```python
from build123d import *

# Parameters (mm, degrees)
SKETCH1_W                        = 12.7
SKETCH1_H                        = 12.7
BOSS_EXTRUDE1_DEPTH              = 72
F_10_24_TAPPED_HOLE1_D           = 3.7973
F_10_24_TAPPED_HOLE2_D           = 3.7973
M6X1_0_TAPPED_HOLE2_D            = 5
M6X1_0_TAPPED_HOLE2_DEPTH        = 20.32
M6X1_0_TAPPED_HOLE2_CSINK_D      = 6.05
M6X1_0_TAPPED_HOLE2_CSINK_ANGLE  = 90
M6X1_0_TAPPED_HOLE2_TIP          = 1.502151548
F_10_24_TAPPED_HOLE3_D           = 3.7973
F_10_24_TAPPED_HOLE3_DEPTH       = 20.574
F_10_24_TAPPED_HOLE3_CSINK_D     = 5.0673
F_10_24_TAPPED_HOLE3_CSINK_ANGLE = 90
F_10_24_TAPPED_HOLE3_TIP         = 1.140824014
LPATTERN1_COUNT                  = 2
LPATTERN1_PITCH                  = 24
LPATTERN2_COUNT                  = 2
LPATTERN2_PITCH                  = 24


with BuildPart() as part:
    # Sketch1 → Boss-Extrude1 (new body)
    with BuildSketch(Plane(origin=(0, 0, 0), x_dir=(0, 0, -1), z_dir=(1, 0, 0))):
        Rectangle(SKETCH1_W, SKETCH1_H)
    extrude(amount=BOSS_EXTRUDE1_DEPTH)

    # #10-24 Tapped Hole1 (through all)
    with Locations(Plane.XY.offset(6.35)):
        with Locations((24, 0)):
            f_10_24_tapped_hole1 = Hole(F_10_24_TAPPED_HOLE1_D / 2)

    # #10-24 Tapped Hole2 (through all)
    with Locations(Plane(origin=(0, 6.35, 0), x_dir=(1, 0, 0), z_dir=(0, 1, 0))):
        with Locations((24, 0)):
            f_10_24_tapped_hole2 = Hole(F_10_24_TAPPED_HOLE2_D / 2)

    # M6x1.0 Tapped Hole2
    with Locations(Plane.ZY):
        with Locations((0, 0)):
            CounterSinkHole(M6X1_0_TAPPED_HOLE2_D / 2, M6X1_0_TAPPED_HOLE2_CSINK_D / 2, depth=M6X1_0_TAPPED_HOLE2_DEPTH, counter_sink_angle=M6X1_0_TAPPED_HOLE2_CSINK_ANGLE)
            with Locations((0, 0, -(M6X1_0_TAPPED_HOLE2_DEPTH + M6X1_0_TAPPED_HOLE2_TIP / 2))):  # 118° drill point
                Cone(0, M6X1_0_TAPPED_HOLE2_D / 2, M6X1_0_TAPPED_HOLE2_TIP, mode=Mode.SUBTRACT)

    # #10-24 Tapped Hole3
    with Locations(Plane(origin=(72, 0, 0), x_dir=(0, 0, -1), z_dir=(1, 0, 0))):
        with Locations((0, 0)):
            CounterSinkHole(F_10_24_TAPPED_HOLE3_D / 2, F_10_24_TAPPED_HOLE3_CSINK_D / 2, depth=F_10_24_TAPPED_HOLE3_DEPTH, counter_sink_angle=F_10_24_TAPPED_HOLE3_CSINK_ANGLE)
            with Locations((0, 0, -(F_10_24_TAPPED_HOLE3_DEPTH + F_10_24_TAPPED_HOLE3_TIP / 2))):  # 118° drill point
                Cone(0, F_10_24_TAPPED_HOLE3_D / 2, F_10_24_TAPPED_HOLE3_TIP, mode=Mode.SUBTRACT)

    # LPattern1: #10-24 Tapped Hole1 ×2
    with Locations(*[(i * LPATTERN1_PITCH, 0, 0) for i in range(1, LPATTERN1_COUNT)]):
        add(f_10_24_tapped_hole1, mode=Mode.SUBTRACT)

    # LPattern2: #10-24 Tapped Hole2 ×2
    with Locations(*[(i * LPATTERN2_PITCH, 0, 0) for i in range(1, LPATTERN2_COUNT)]):
        add(f_10_24_tapped_hole2, mode=Mode.SUBTRACT)


solid = part.part
```
Read the model definition and answer for the solid it produces. Units are mm, in the model's axes. A direction names the side the tool comes from. Round coordinates to 2 decimals unless told otherwise and drop trailing zeros. Write each loop counter-clockwise with the first axis right and the second up, starting at its lowest first coordinate (ties: lowest second). Pieces come first, ordered by that corner, then holes. Notation, with made-up numbers: (87, 78) - (123, 78) arc R17 cw to (123, 94) - close; hole circle Ø10 at (82.5, 56). An arc over 180 degrees is marked (long way). One line per item, written item: value.
Q1. Straight lines are drawn through the part: line 1 (Z direction, x = 5.5, y = 0); line 2 (X direction, y = -4, z = -1); line 3 (Z direction, x = 61, y = 0). For each, find the intervals that lie inside material, in ascending order. Write a range as from..to.
The answers:
line 1: z = -6.35..-2.5, 2.5..6.35
line 2: x = 0..22.39, 25.61..46.39, 49.61..72
line 3: z = -6.35..-1.9, 1.9..6.35
Q2. Find section D-D (x = 8). Determine the outline of the cut face in (y, z).
The answers:
outline: (-6.35, -6.35) - (6.35, -6.35) - (6.35, 6.35) - (-6.35, 6.35) - close; hole circle Ø5 at (0, 0)
Q3. Find section A-A (x = 24). Determine the outline of the cut face in (y, z).
The answers:
outline: (-6.35, -6.35) - (-1.9, -6.35) - (-1.9, -1.9) - (-6.35, -1.9) - close; (-6.35, 1.9) - (-1.9, 1.9) - (-1.9, 6.35) - (-6.35, 6.35) - close; (1.9, -6.35) - (6.35, -6.35) - (6.35, -1.9) - (1.9, -1.9) - close; (1.9, 1.9) - (6.35, 1.9) - (6.35, 6.35) - (1.9, 6.35) - close
Q4. For a pull along X with two mould halves and no side action, classify faces 1 (the cylindrical face through (46.2, 0.6, -3.9)), 2 (the conical face through (50.48, 0.1, -0.31)), 3 (the flat face through (35, 0, 6.35)) as pulls with the +X half, pulls with the -X half, needs draft (parallel to the pull), parting line crosses it, or undercut.
The answers:
face 1: undercut
face 2: pulls with the +X half
face 3: needs draft
Q5. Each of these flat-tipped pins is pushed along its axis until it touches: P1, Ø2.5, axis at x = 48, y = 0, coming from the +Z side; P2, Ø6, axis at y = 0, z = 0, coming from the -X side (3 decimals); P3, Ø4.5, axis at y = 0, z = 0, coming from the -X side. Where does it stop, or does it pass through?
The answers:
P1: passes through
P2: stops at x = 0.025
P3: stops at x = 20.47
Q6. Find section B-B (z = 4.25). Determine the outline of the cut face in (x, y).
The answers:
outline: (0, -6.35) - (72, -6.35) - (72, 6.35) - (0, 6.35) - close; hole circle Ø3.8 at (24, 0); hole circle Ø3.8 at (48, 0)
Q7. Which of the six approach directions +Z, -Z, +X, -X, +Y, -Y give full straight-line access (tool end or side, diameter ignored) to faces 4 (the cylindrical face through (61.3, 0.6, 1.8)), 5 (the flat face through (72, 0, -3)), 6 (the cylindrical face through (10.56, -2.44, 0.54))?
The answers:
face 4: +X
face 5: +Z, -Z, +X, +Y, -Y
face 6: -X
